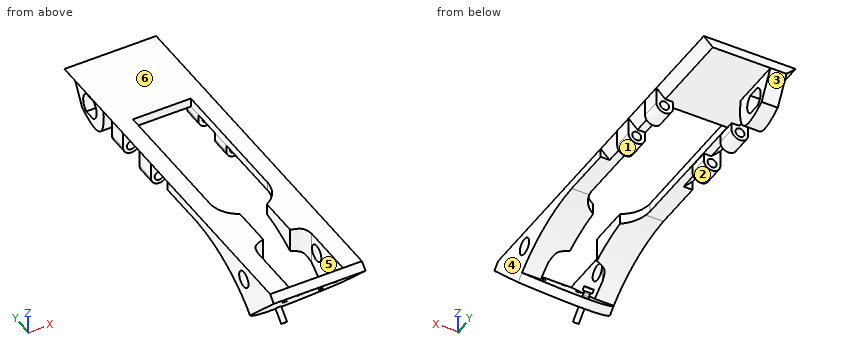
```python
from build123d import *

# Parameters (mm, degrees)
SKETCH1_R           = 2.5
BOSS_EXTRUDE1_DEPTH = 200
SKETCH4_W           = 8.702747253
SKETCH4_H           = 30
SKETCH4_H_2         = 16
CUT_EXTRUDE4_DEPTH  = 207.854454345
CHAMFER2_SIZE       = 5
CHAMFER2_SIZE_2     = 5.019354123
BOSS_EXTRUDE2_DEPTH = 51
CUT_EXTRUDE5_DEPTH  = 203.964396132
SKETCH8_R           = 4.5
CUT_EXTRUDE6_DEPTH  = 208.714458096
BOSS_EXTRUDE3_DEPTH = 5
BOSS_EXTRUDE4_START = -13
SKETCH10_R          = 1.5
BOSS_EXTRUDE4_DEPTH = 16
CHAMFER11_SIZE      = 5
SKETCH11_R          = 2.5
BOSS_EXTRUDE5_DEPTH = 2
FILLET1_R           = 1
BOSS_EXTRUDE6_START = -5
BOSS_EXTRUDE6_DEPTH = 9
SKETCH14_R          = 1.5
CUT_EXTRUDE7_DEPTH  = 10
CUT_EXTRUDE8_START  = -84
CUT_EXTRUDE8_DEPTH  = 16


# Some blends are built 0.0001 mm under size
with BuildPart() as part:
    # Sketch1 → Boss-Extrude1 (new body)
    with BuildSketch(Plane(origin=(0, 0, 0), x_dir=(1, 0, 0), z_dir=(0, 1, 0))):
        with BuildLine():
            Line((-25.5, 5), (-25.5, 9.107142857))
            ThreePointArc((-25.5, 9.107142857), (-20.904395604, 13.702747253), (-16.308791209, 9.107142857))
            Line((-16.308791209, 9.107142857), (-16.308791209, 5))
            Line((-16.308791209, 5), (16.308791209, 5))
            Line((16.308791209, 5), (16.308791209, 9.107142857))
            ThreePointArc((16.308791209, 9.107142857), (20.904395604, 13.702747253), (25.5, 9.107142857))
            Line((25.5, 9.107142857), (25.5, 5))
            Line((25.5, 5), (25.5, 0))
            Line((25.5, 0), (-25.5, 0))
            Line((-25.5, 0), (-25.5, 5))
        make_face()
        with Locations(Location((-20.96043956, 9.107142857, 0), (0, 0, 270))):
            Circle(SKETCH1_R, mode=Mode.SUBTRACT)
        with Locations(Location((20.96043956, 9.107142857, 0), (0, 0, 90))):
            Circle(SKETCH1_R, mode=Mode.SUBTRACT)
    extrude(amount=BOSS_EXTRUDE1_DEPTH)

    # Sketch4 → Cut-Extrude4 (cut, through all)
    with BuildSketch(Plane(origin=(25.5, 0, 0), x_dir=(0, 0, -1), z_dir=(1, 0, 0))):
        with Locations((9.351373626, 185)):
            Rectangle(SKETCH4_W, SKETCH4_H)
        with Locations((9.351373626, 162)):
            Rectangle(SKETCH4_W, SKETCH4_H_2)
        with Locations((9.351373626, 135)):
            Rectangle(SKETCH4_W, SKETCH4_H_2)
        with Locations((9.351373626, 108)):
            Rectangle(SKETCH4_W, SKETCH4_H_2)
        Polygon((5, 100), (5, 116), (4.553571429, 0), (13.702747253, 0), (13.702747253, 100), align=None)
    extrude(amount=-CUT_EXTRUDE4_DEPTH, mode=Mode.SUBTRACT)

    # Chamfer2
    # the kernel refuses this chamfer: 5.019354123, 5 mm, written as the material it takes off along each edge
    with BuildSketch(Plane(origin=(38.409512828, 0, -4.553571429), x_dir=(0, 0.9995054486557426, -0.03144611434633402), z_dir=(-1, 0, 0))) as chamfer2_piece_1:
        Polygon((CHAMFER2_SIZE * 0.999619067011, -CHAMFER2_SIZE * 0.0275992910832), (-CHAMFER2_SIZE_2 * 0.0314461143481, -CHAMFER2_SIZE_2 * 0.999505448712), (0, 0), align=None)
    extrude(amount=76.819025655, mode=Mode.SUBTRACT)

    # Sketch7 → Boss-Extrude2 (add, through all)
    with BuildSketch(Plane.ZY.offset(25.5)):
        with BuildLine():
            Line((-4.572813897, 4.999962973), (-23.330153181, 23.613479688))
            add(Edge.make_bspline(
                [(-23.330153181, 23.613479688), (-6.160592573, 44.077045925), (-4.829970579, 71.819555154)],
                knots=[0, 0, 0, 1, 1, 1], degree=2))
            Line((-4.829970579, 71.819555154), (-4.572813897, 4.999962973))
        make_face()
    extrude(amount=-BOSS_EXTRUDE2_DEPTH)

    # Sketch5 → Cut-Extrude5 (cut, through all)
    with BuildSketch(Plane.XY):
        with BuildLine():
            Line((-16.096845958, 150), (-16.096845958, 75.462211289))
            ThreePointArc((-16.096845958, 75.462211289), (-13.78105211, 67.144095363), (-7.5, 61.219372745))
            Line((-7.5, 61.219372745), (-7.5, 38.659982869))
            add(Edge.make_bspline(
                [(-7.5, 38.659982869), (-9.795642151, 38.017223862), (-13.947085411, 36.854857355), (-14.674726057, 32.692610158), (-15, 30.831979414)],
                knots=[0, 0, 0, 0, 0.552974474, 1, 1, 1, 1], degree=3))
            Line((-15, 30.831979414), (-15, 0))
            Line((-15, 0), (15, 0))
            Line((15, 0), (15, 30.831979414))
            add(Edge.make_bspline(
                [(7.5, 38.659982869), (9.795642151, 38.017223862), (13.947085411, 36.854857355), (14.674726057, 32.692610158), (15, 30.831979414)],
                knots=[0, 0, 0, 0, 0.552974474, 1, 1, 1, 1], degree=3))
            Line((7.5, 38.659982869), (7.5, 61.219372745))
            ThreePointArc((7.5, 61.219372745), (13.78105211, 67.144095363), (16.096845958, 75.462211289))
            Line((16.096845958, 75.462211289), (16.096845958, 150))
            Line((16.096845958, 150), (-16.096845958, 150))
        make_face()
    extrude(amount=-CUT_EXTRUDE5_DEPTH, mode=Mode.SUBTRACT)

    # Sketch8 → Cut-Extrude6 (cut, through all)
    with BuildSketch(Plane.ZY.offset(25.5)):
        with Locations((-8.727098944, 26.028021636)):
            Circle(SKETCH8_R)
    extrude(amount=-CUT_EXTRUDE6_DEPTH, mode=Mode.SUBTRACT)

    # Sketch9 → Boss-Extrude3 (add)
    with BuildSketch(Plane(origin=(0, 0.232884449, 0.231098799), x_dir=(1, 0, 0), z_dir=(0, -0.7098228406915363, -0.7043802487524746))):
        with BuildLine():
            Line((-25.5, -0.325572503), (-25.5, -33.193144301))
            add(Edge.make_bspline(
                [(-25.5, -33.193144301), (0, -92.295534264), (25.5, -33.193144301)],
                knots=[0, 0, 0, 1, 1, 1], degree=2))
            Line((25.5, -33.193144301), (25.5, -0.325572503))
            Line((25.5, -0.325572503), (-25.5, -0.325572503))
        make_face()
    extrude(amount=BOSS_EXTRUDE3_DEPTH)

    # Sketch10 → Boss-Extrude4 (add)
    with BuildSketch(Plane(origin=(0, 0.232884449, 0.231098799), x_dir=(1, 0, 0), z_dir=(0, 0.7098228406915363, 0.7043802487524746)).offset(BOSS_EXTRUDE4_START)):
        with Locations(Location((0, 57.339451639, 0), (0, 0, 270))):
            Circle(SKETCH10_R)
    extrude(amount=BOSS_EXTRUDE4_DEPTH)

    # Chamfer11
    chamfer11_edges = [part.edges().sort_by_distance(p)[0] for p in [
        (25.5, 135, -5),
        (25.5, 177, -5),
        (-25.5, 135, -5),
        (-25.5, 177, -5),
    ]]
    chamfer(chamfer11_edges, length=CHAMFER11_SIZE - 0.0001)  # a hair under: the kernel refuses the full size

    # Sketch11 → Boss-Extrude5 (add)
    with BuildSketch(Plane(origin=(0, 2.362352971, 2.344239545), x_dir=(1, 0, 0), z_dir=(0, 0.7098228406915363, 0.7043802487524746))):
        with Locations(Location((0, 57.339451639, 0), (0, 0, 270))):
            Circle(SKETCH11_R)
    extrude(amount=BOSS_EXTRUDE5_DEPTH)

    # Fillet1
    fillet1_edges = [part.edges().sort_by_distance(p)[0] for p in [
        (0, 41.678232031, -41.534487908),
        (0, 43.807700553, -39.421347162),
    ]]
    fillet(fillet1_edges, radius=FILLET1_R - 0.0001)  # a hair under: the kernel refuses the full size

    # Sketch13 → Boss-Extrude6 (add)
    with BuildSketch(Plane.ZY.offset(25.5).offset(BOSS_EXTRUDE6_START)):
        with BuildLine():
            Line((-5, 171), (-5, 200))
            Line((-5, 200), (-20.018483641, 191.448737676))
            add(Edge.make_bspline(
                [(-5, 171), (-33.25422997, 167.518026698), (-20.018483641, 191.448737676)],
                knots=[0, 0, 0, 1, 1, 1], degree=2))
        make_face()
        with BuildLine():
            Line((-19.5, 180.535898385), (-19.5, 187.464101615))
            ThreePointArc((-19.5, 187.464101615), (-14, 190.5), (-8.5, 187.464101615))
            Line((-8.5, 187.464101615), (-8.5, 180.535898385))
            ThreePointArc((-8.5, 180.535898385), (-14, 177.5), (-19.5, 180.535898385))
        make_face(mode=Mode.SUBTRACT)
    extrude(amount=-BOSS_EXTRUDE6_DEPTH)

    # Sketch14 → Cut-Extrude7 (cut)
    with BuildSketch(Plane(origin=(0, -3.316229755, -3.290802445), x_dir=(1, 0, 0), z_dir=(0, -0.7098228406915363, -0.7043802487524746))):
        with Locations(Location((-10, -3.325572503, 0), (0, 0, 270))):
            Circle(SKETCH14_R)
        with Locations(Location((-10, -23.325572503, 0), (0, 0, 270))):
            Circle(SKETCH14_R)
        with Locations(Location((10, -23.325572503, 0), (0, 0, 90))):
            Circle(SKETCH14_R)
        with Locations(Location((10, -3.325572503, 0), (0, 0, 90))):
            Circle(SKETCH14_R)
    extrude(amount=-CUT_EXTRUDE7_DEPTH, mode=Mode.SUBTRACT)

    # Sketch15 → Cut-Extrude8 (cut)
    with BuildSketch(Plane(origin=(0, 200, 0), x_dir=(1, 0, 0), z_dir=(0, 1, 0)).offset(CUT_EXTRUDE8_START)):
        Polygon((25.5, 0), (20.5, 5), (25.5, 5), align=None)
        Polygon((-20.5, 5), (-25.5, 0), (-25.5, 5), align=None)
    extrude(amount=-CUT_EXTRUDE8_DEPTH, mode=Mode.SUBTRACT)


solid = part.part
```
Model file for the job. Use its own axes, mm. Face numbers are marked on the shaded views. A direction names the side the tool comes from. Coordinates: 2 decimals unless noted, no trailing zeros. Write each loop counter-clockwise with the first axis right and the second up, starting at its lowest first coordinate (ties: lowest second). Pieces come first, ordered by that corner, then holes. Notation, with made-up numbers: (-6.5, -16) - (22.5, -16) arc R11 cw to (22.5, 2) - close; hole circle Ø5 at (78.5, 83.25). An arc over 180 degrees is marked (long way). Use a Markdown table: item, result. Add a question column.
Item 1: 3-axis set-ups, long thin cutter, end or side, ignore diameter. For the marked faces 1, 2 and 3: which of +Z, -Z, +X, -X, +Y, -Y reach the whole face in a straight line?
Item 2: Two-plate mould, pull along X, no slides. Class the marked faces 4, 5 and 6: pulls with the +X half, pulls with the -X half, needs draft (parallel to the pull), parting line crosses it, or undercut.
Item 3: Drill centre lines: line 1 along Z through (x, y) = (-2, 169); line 2 along X through (y, z) = (42.5, -8); line 3 along X through (y, z) = (125, -4). Where is each one in solid material? Low to high.
Item 4: Band-saw the part on B-B, the plane y = 95.5. Write the cut outline in (x, z).
Item 5: Drop flat-ended pins along their axis: pin 1 (5 mm diameter, centred on y = 128.5, z = -5.5, fed in from +X); pin 2 (10 mm diameter, centred on x = 20, z = -32.5, fed in from +Y); pin 3 (3 mm diameter, centred on x = 22, z = -9, fed in from +Y); pin 4 (7.5 mm diameter, centred on x = -22.5, z = -10, fed in from +Y). Give the stop position or say it passes through.
A:
| question | item | result |
|---|---|---|
| 1 | face 1 | -Z, +Y |
| 1 | face 2 | -Z |
| 1 | face 3 | -Z, +X, -X, +Y |
| 2 | face 4 | pulls with the +X half |
| 2 | face 5 | undercut |
| 2 | face 6 | needs draft |
| 3 | line 1 | z = -5 to 0 |
| 3 | line 2 | x = -25.5 to -7.5, 7.5 to 25.5 |
| 3 | line 3 | x = -25.5 to -16.1, 16.1 to 25.5 |
| 4 | outline | (-25.5, -4.92) - (-16.1, -4.92) - (-16.1, 0) - (-25.5, 0) - close; (16.1, -4.92) - (25.5, -4.92) - (25.5, 0) - (16.1, 0) - close |
| 5 | pin 1 | stops at x = 25.5 |
| 5 | pin 2 | stops at y = 35.98 |
| 5 | pin 3 | stops at y = 154 |
| 5 | pin 4 | stops at y = 198.96 |
